Study the drawing (mm; zero at the part's minimum x, y, z) and answer. A direction names the side the tool comes from. Give positions to 0.01 mm unless a question says otherwise; leave off trailing zeros. Write each loop counter-clockwise with the first axis right and the second up, starting at its lowest first coordinate (ties: lowest second). Pieces come first, ordered by that corner, then holes. Notation, with made-up numbers: (41.25, -0.5) - (60.25, -0.5) arc R15 cw to (60.25, 17.5) - close; hole circle Ø5 at (6, 10). An arc over 180 degrees is marked (long way). Return JSON: item names as keys, results as strings.
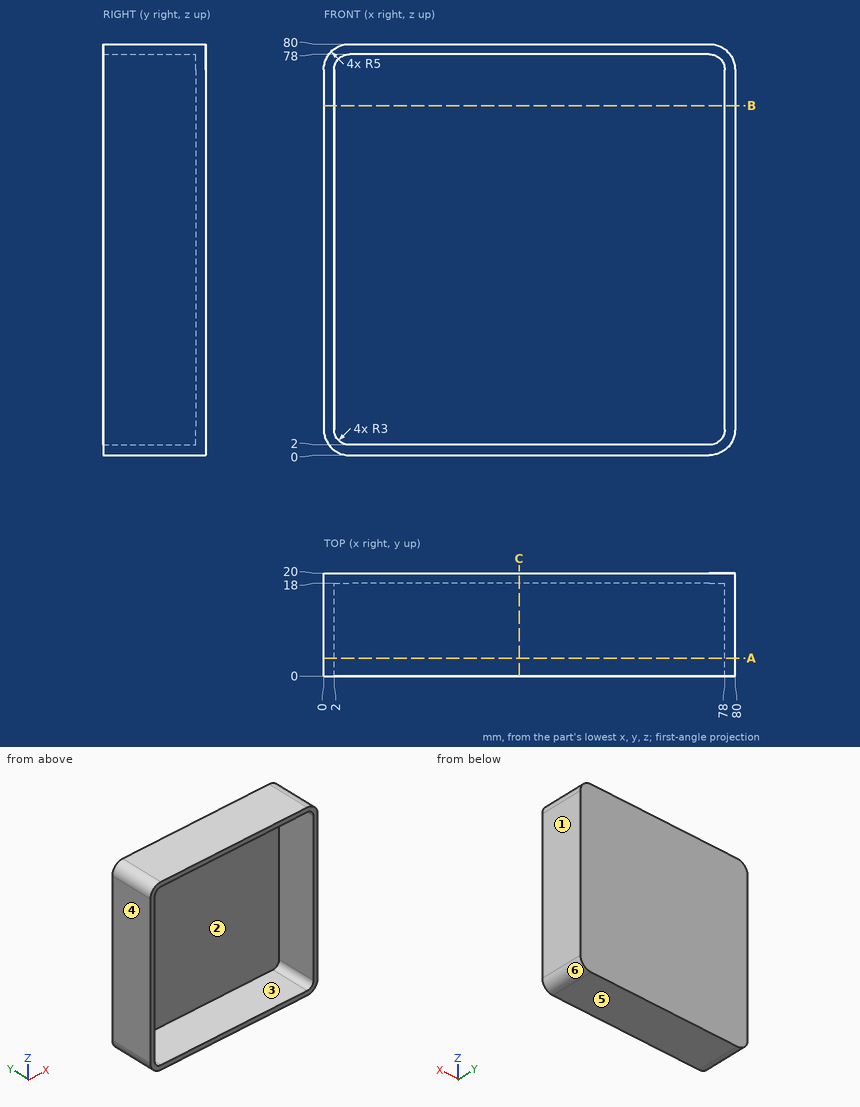
Item 1: Flat-ended cylindrical pins translate along their axes: P1, Ø5.5, axis at y = 7, z = 28.5, coming from the -X side; P2, Ø4, axis at x = 67.5, z = 26, coming from the -Y side. Find the tip coordinate at first contact, or state that the pin passes through.
Answer below:
{"P1": "stops at x = 0", "P2": "stops at y = 18"}
Item 2: A cutting plane is placed at A-A on y = 3.5. Determine the outline of the cut face in (x, z), then the cut area to 3 significant figures.
Answer below:
{"outline": "(0, 5) arc R5 ccw to (5, 0) - (75, 0) arc R5 ccw to (80, 5) - (80, 75) arc R5 ccw to (75, 80) - (5, 80) arc R5 ccw to (0, 75) - close; hole (2, 5) arc R3 ccw to (5, 2) - (75, 2) arc R3 ccw to (78, 5) - (78, 75) arc R3 ccw to (75, 78) - (5, 78) arc R3 ccw to (2, 75) - close", "area": "610 mm²"}
Item 3: Consider L1, parallel to X at y = 15.5, z = 9.5; L2, parallel to Y at x = 35, z = 55.5. Determine where each line is inside the solid, lowest interval first.
Answer below:
{"L1": "x = 0 to 2, 78 to 80", "L2": "y = 18 to 20"}
Item 4: For the marked faces 1 and 2, determine the directions among +Z, -Z, +X, -X, +Y, -Y from which every point of the face is accessible in a straight line to the end or side of a thin tool.
Answer below:
{"face 1": "+Z, -Z, +X, +Y, -Y", "face 2": "-Y"}
Item 5: A cutting plane is placed at C-C on x = 38. Determine the outline of the cut face in (y, z).
Answer below:
{"outline": "(0, 0) - (20, 0) - (20, 80) - (0, 80) - (0, 78) - (18, 78) - (18, 2) - (0, 2) - close"}
Item 6: A cutting plane is placed at B-B on z = 68. Determine the outline of the cut face in (x, y), then the cut area to 3 significant figures.
Answer below:
{"outline": "(0, 0) - (2, 0) - (2, 18) - (78, 18) - (78, 0) - (80, 0) - (80, 20) - (0, 20) - close", "area": "232 mm²"}
Item 7: The mould has two halves that part along X. Classify the marked faces 3, 4, 5 and 6: +X half, -X half, draft (parallel to the pull), parting line (faces both ways), or undercut.
Answer below:
{"face 3": "undercut", "face 4": "-X half", "face 5": "draft", "face 6": "+X half"}
